```python
from build123d import *

# Parameters (mm, degrees)
SKETCH2_R           = 12.7
SKETCH3_W           = 50.8
SKETCH3_H           = 50.8
BOSS_EXTRUDE1_DEPTH = 50.8
SKETCH4_R           = 12.7
BOSS_EXTRUDE2_DEPTH = 626.8
SKETCH5_R           = 12.7
BOSS_EXTRUDE3_DEPTH = 625.8


with BuildPart() as part:
    # Sweep1: sweep along a path in Sketch1
    with BuildLine(Plane.XY) as sweep1_path:
        Line((0, 0), (0, 203.2))
        ThreePointArc((0, 203.2), (37.197438789, 293.002561211), (127, 330.2))
        Line((127, 330.2), (508, 330.2))
        ThreePointArc((508, 330.2), (597.802561211, 293.002561211), (635, 203.2))
        Line((635, 203.2), (635, 0))
    # Sketch2 → Sweep1 (sweep)
    with BuildSketch(Plane(origin=(0, 0, 0), x_dir=(1, 0, 0), z_dir=(0, 1, 0))):
        Circle(SKETCH2_R)
    sweep(path=sweep1_path.line)

    # Sketch3 → Boss-Extrude1 (add)
    with BuildSketch(Plane.XZ):
        Rectangle(SKETCH3_W, SKETCH3_H)
        with Locations((635, 0)):
            Rectangle(SKETCH3_W, SKETCH3_H)
    extrude(amount=BOSS_EXTRUDE1_DEPTH)

    # Sketch4 → Boss-Extrude2 (add)
    with BuildSketch(Plane(origin=(0, 0, 0), x_dir=(0, 0, -1), z_dir=(1, 0, 0))):
        with Locations((0, 203.2)):
            Circle(SKETCH4_R)
    extrude(amount=BOSS_EXTRUDE2_DEPTH)

    # Sketch5 → Boss-Extrude3 (add)
    with BuildSketch(Plane(origin=(0, 0, 0), x_dir=(0, 0, -1), z_dir=(1, 0, 0))):
        with Locations((0, 82.09908093)):
            Circle(SKETCH5_R)
    extrude(amount=BOSS_EXTRUDE3_DEPTH)


solid = part.part
```
Here's how the part is built. I have some questions about the finished solid (model axes, mm). A direction names the side the tool comes from. Coordinates: 2 decimals unless noted, no trailing zeros. Loops run counter-clockwise (first coordinate to the right, second up) from the corner with the lowest first, then second, coordinate; pieces in that order, holes last. Notation, with made-up numbers: (-5, 31) - (22, 31) arc R24 ccw to (22, 60) - close; hole circle Ø3 at (17.25, -15.75). An arc over 180 degrees is marked (long way). Return JSON: item names as keys, results as strings. Group by question number.
Item 1: If we section it at C-C on x = 210: Write out the boundary of the cut face in (y, z).
Item 2: If we section it at B-B on z = 0: Write out the boundary of the cut face in (x, y).
Item 3: We'd pull the mould along Y, two halves only. Please class faces 1 (the face through (635, -25, -25.4)), 2 (the face through (629, 0, 12)), 3 (the face through (635, -50.8, 0)): +Y half, -Y half, draft (parallel to the pull), parting line (faces both ways), or undercut.
Item 4: Will these pins go through, and if not, where does the flat tip stop? P1, Ø12, axis at y = 149, z = 2.5, coming from the -X side; P2, Ø1.5, axis at x = 339.5, y = 82.5, coming from the -Z side; P3, Ø2.5, axis at y = 205.5, z = 11, coming from the +X side.
Item 5: If we section it at A-A on y = 146: Write out the boundary of the cut face in (x, z), and give its area (3 significant figures).
Item 6: If we section it at D-D on x = 594: State how many separate pieces and enclosed holes the cut face has, and give its area (3 significant figures).
Item 7: I need wall thicknesses on line 1 (X direction, y = -13, z = 14.5); line 2 (Y direction, x = 548.5, z = -8.5); line 3 (Y direction, x = 248, z = 5.5). Which ranges of each line are inside material? Lowest first, please. Write a range as from..to.
Item 8: On a 3-axis mill with a long thin cutter (end or side, diameter ignored), from which of +Z, -Z, +X, -X, +Y, -Y can I reach the whole of each face in a straight line? I mean faces 4 (the face through (0, -25, -25.4)), 5 (the face through (25.4, -25, 0)), 6 (the face through (647.688, 100.178, -0.558)). Say none if no direction works.
Calculated:
{
 "1": {"outline": "circle Ø25.4 at (82.1, 0); circle Ø25.4 at (203.2, 0); circle Ø25.4 at (330.2, 0)"},
 "2": {"outline": "(-25.4, -50.8) - (25.4, -50.8) - (25.4, 0) - (12.7, 0) - (12.7, 69.4) - (622.3, 69.4) - (622.3, 0) - (609.6, 0) - (609.6, -50.8) - (660.4, -50.8) - (660.4, 0) - (647.7, 0) - (647.7, 203.2) arc R139.7 ccw to (508, 342.9) - (127, 342.9) arc R139.7 ccw to (-12.7, 203.2) - (-12.7, 0) - (-25.4, 0) - close; hole (12.7, 94.8) - (622.3, 94.8) - (622.3, 190.5) - (12.7, 190.5) - close; hole (13.41, 215.9) - (621.59, 215.9) arc R114.3 ccw to (508, 317.5) - (127, 317.5) arc R114.3 ccw to start"},
 "3": {"face 1": "draft", "face 2": "undercut", "face 3": "-Y half"},
 "4": {"P1": "stops at x = -12.7", "P2": "stops at z = -12.7", "P3": "stops at x = 643.12"},
 "5": {"outline": "circle Ø25.4 at (0, 0); circle Ø25.4 at (635, 0)", "area": "1,010 mm^2"},
 "6": {"separate pieces": "3", "enclosed holes": "0", "area": "1,710 mm^2"},
 "7": {"line 1": "x = -25.4..25.4, 609.6..660.4", "line 2": "y = 72.66..91.54, 193.76..212.64, 313.57..333.49", "line 3": "y = 70.65..93.55, 191.75..214.65, 318.75..341.65"},
 "8": {"face 4": "-Z, +X, -X, +Y, -Y", "face 5": "+Z, -Z, -Y", "face 6": "none"}
}
